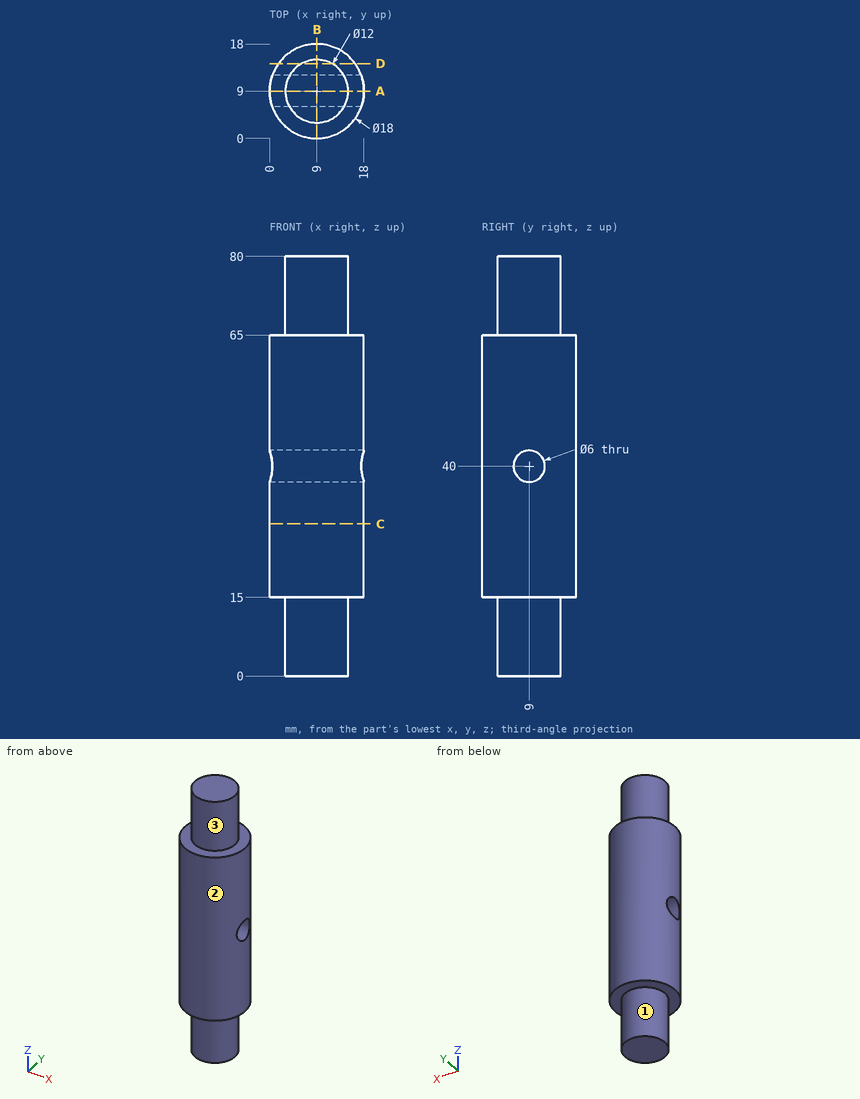
Print and shaded views of the part. All mm, measured from the part's lowest x, y and z. A direction names the side the tool comes from. Round coordinates to 2 decimals unless told otherwise and drop trailing zeros. Write each loop counter-clockwise with the first axis right and the second up, starting at its lowest first coordinate (ties: lowest second). Pieces come first, ordered by that corner, then holes.
Item 1: Cut at C-C, the plane z = 29. Give the cut face in (x, y).
Results:
outline: circle Ø18 at (9, 9)
Item 2: Cut at B-B, the plane x = 9. Give the cut face in (y, z).
Results:
outline: (0, 15) - (3, 15) - (3, 0) - (15, 0) - (15, 15) - (18, 15) - (18, 65) - (15, 65) - (15, 80) - (3, 80) - (3, 65) - (0, 65) - close; hole circle Ø6 at (9, 40)
Item 3: Cut at D-D, the plane y = 14.25. Give the cut face in (x, z), plus the area to 3 significant figures.
Results:
outline: (1.69, 15) - (6.1, 15) - (6.1, 0) - (11.9, 0) - (11.9, 15) - (16.31, 15) - (16.31, 65) - (11.9, 65) - (11.9, 80) - (6.1, 80) - (6.1, 65) - (1.69, 65) - close
area: 905 mm2
Item 4: Drop flat-ended pins along their axis: pin 1 Ø4 at (y, z) = (16, 42) entering from +X; pin 2 Ø2 at (x, z) = (11.5, 8.5) entering from +Y; pin 3 Ø1.5 at (x, z) = (8, 11) entering from +Y. Give the stop position or say it passes through.
Results:
pin 1: stops at x = 16.48
pin 2: stops at y = 14.81
pin 3: stops at y = 14.99
Item 5: Which spindle directions (+Z, -Z, +X, -X, +Y, -Y) get a long thin tool onto all of the face, cutting with end or side? Do the marked faces 1, 2 and 3. Say none if no direction does.
Results:
face 1: -Z
face 2: +Z, -Z
face 3: +Z
Item 6: Probe L1, parallel to Z at x = 8, y = 7.25; L2, parallel to Y at x = 3.5, z = 37.5; L3, parallel to Y at x = 9.25, z = 40. List the from-to ranges inside material, lowest first.
Results:
L1: z = 0 to 37.56, 42.44 to 80
L2: y = 1.88 to 7.34, 10.66 to 16.12
L3: y = 0 to 6, 12 to 18
Item 7: Cut at A-A, the plane y = 9. Give the cut face in (x, z).
Results:
outline: (0, 15) - (3, 15) - (3, 0) - (15, 0) - (15, 15) - (18, 15) - (18, 37) - (0, 37) - close; (0, 43) - (18, 43) - (18, 65) - (15, 65) - (15, 80) - (3, 80) - (3, 65) - (0, 65) - close
